Here's how the part is built. I have some questions about the finished solid (model axes, mm). Face numbers are marked on the shaded views. A direction names the side the tool comes from. Round coordinates to 2 decimals unless told otherwise and drop trailing zeros. Write each loop counter-clockwise with the first axis right and the second up, starting at its lowest first coordinate (ties: lowest second). Pieces come first, ordered by that corner, then holes. Notation, with made-up numbers: M 20,-15.75 L 42,-15.75 A13 ccw 42,-0.75 Z; hole C 60,7.5 d7. An arc over 180 degrees is marked long. Use one line per item in the form item = value. Start each with the question number.
Q1. For the marked faces 5 and 6, which set-ups out of +Z, -Z, +X, -X, +Y, -Y let a thin tool reach every point of the face, with its end or its side?
Q2. I'm going to push flat-ended pins straight in: pin 1 Ø8 at (y, z) = (4.5, 1) entering from +X; pin 2 Ø0.6 at (x, y) = (-9, 3) entering from -Z. Where does each tip first touch, or does it pass through?
Q3. We'd pull the mould along X, two halves only. Please class the marked faces 1, 2, 3 and 4: +X half, -X half, draft (parallel to the pull), parting line (faces both ways), or undercut.
Q4. I need wall thicknesses on line 1 along Z through (x, y) = (-9, 0.75). Which ranges of the line are inside material? Lowest first, please. Write a range as from..to.
Q5. I want a section at A-A on x = 6. List the corners of the cut face in (y, z) for me.
Q6. I want a section at B-B on y = 0. List the corners of the cut face in (x, z) for me.
Q7. I want a section at D-D on y = 8. List the corners of the cut face in (x, z) for me, and give its area (3 significant figures).
Q8. I want a section at C-C on z = 4.25. List the corners of the cut face in (x, y) for me, and give its area (3 significant figures).
```python
from build123d import *

# Parameters (mm, degrees)
SKETCH1_W           = 20
SKETCH1_H           = 20
SKETCH1_W_2         = 16
SKETCH1_H_2         = 16
BOSS_EXTRUDE1_DEPTH = 10
SKETCH2_W           = 14
SKETCH2_H           = 14
CUT_EXTRUDE1_DEPTH  = 21
SKETCH3_W           = 14
SKETCH3_H           = 14
CUT_EXTRUDE2_DEPTH  = 21
SKETCH4_W           = 2
SKETCH4_H           = 14
BOSS_EXTRUDE2_DEPTH = 14
SKETCH5_R           = 7.5
BOSS_EXTRUDE3_DEPTH = 5


with BuildPart() as part:
    # Sketch1 → Boss-Extrude1 (new body, symmetric)
    with BuildSketch(Plane(origin=(0, 0, 0), x_dir=(1, 0, 0), z_dir=(0, 1, 0))):
        Rectangle(SKETCH1_W, SKETCH1_H)
        Rectangle(SKETCH1_W_2, SKETCH1_H_2, mode=Mode.SUBTRACT)
    extrude(amount=BOSS_EXTRUDE1_DEPTH, both=True)

    # Sketch2 → Cut-Extrude1 (cut, through all)
    with BuildSketch(Plane.XY.offset(10)):
        Rectangle(SKETCH2_W, SKETCH2_H)
    extrude(amount=-CUT_EXTRUDE1_DEPTH, mode=Mode.SUBTRACT)

    # Sketch3 → Cut-Extrude2 (cut, through all)
    with BuildSketch(Plane(origin=(10, 0, 0), x_dir=(0, 0, -1), z_dir=(1, 0, 0))):
        Rectangle(SKETCH3_W, SKETCH3_H)
    extrude(amount=-CUT_EXTRUDE2_DEPTH, mode=Mode.SUBTRACT)

    # Sketch4 → Boss-Extrude2 (add)
    with BuildSketch(Plane(origin=(-7, 0, 0), x_dir=(0, 0, -1), z_dir=(1, 0, 0))):
        with Locations((9, 0)):
            Rectangle(SKETCH4_W, SKETCH4_H)
    extrude(amount=BOSS_EXTRUDE2_DEPTH)

    # Sketch5 → Boss-Extrude3 (add)
    with BuildSketch(Plane(origin=(0, 0, -10), x_dir=(-1, 0, 0), z_dir=(0, 0, -1))):
        Circle(SKETCH5_R)
    extrude(amount=BOSS_EXTRUDE3_DEPTH)


solid = part.part
```
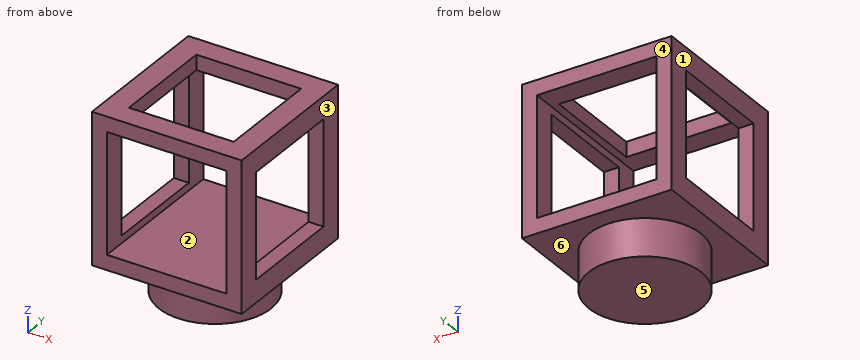
Reported:
q1.face_5 = -Z, +X, -X, +Y, -Y
q1.face_6 = -Z
q2.pin_1 = 10
q2.pin_2 = -10
q3.face_1 = -X half
q3.face_2 = undercut
q3.face_3 = +X half
q3.face_4 = draft
q4.line_1 = -10..-7, 7..10
q5.outline = M -10,-10 L -4.5,-10 L -4.5,-15 L 4.5,-15 L 4.5,-10 L 10,-10 L 10,-8 L -10,-8 Z; M -10,8 L -7,8 L -7,10 L -10,10 Z; M 7,8 L 10,8 L 10,10 L 7,10 Z
q6.outline = M -10,-10 L -7.5,-10 L -7.5,-15 L 7.5,-15 L 7.5,-10 L 10,-10 L 10,-7 L 8,-7 L 8,-8 L -8,-8 L -8,-7 L -10,-7 Z; M -10,7 L -8,7 L -8,8 L -7,8 L -7,10 L -10,10 Z; M 7,8 L 8,8 L 8,7 L 10,7 L 10,10 L 7,10 Z
q7.outline = M -10,-10 L 10,-10 L 10,10 L -10,10 Z; hole M -8,-8 L 8,-8 L 8,8 L -8,8 Z
q7.area = 144 mm^2
q8.outline = M -10,-10 L -8,-10 L -8,-7 L -10,-7 Z; M -10,7 L -8,7 L -8,10 L -10,10 Z; M 8,-10 L 10,-10 L 10,-7 L 8,-7 Z; M 8,7 L 10,7 L 10,10 L 8,10 Z
q8.area = 24.0 mm^2
